Could you check a few things on this model? Use its own coordinates, in mm. A direction names the side the tool comes from. Coordinates: 2 decimals unless noted, no trailing zeros. Loops run counter-clockwise (first coordinate to the right, second up) from the corner with the lowest first, then second, coordinate; pieces in that order, holes last. Notation, with made-up numbers: M 60,80.25 L 111,80.25 A12 ccw 111,88.25 Z; hole C 3,-24 d2. An arc over 180 degrees is marked long. Write each question's results on one line, items separated by ' | '.
```python
from build123d import *

# Parameters (mm, degrees)
F1_DEPTH  = 40
F3_DEPTH  = 10
F4_W      = 20
F4_H      = 20
F5_DEPTH  = 20
F7_DEPTH  = 20
F9_DEPTH  = 20
F11_DEPTH = 20


with BuildPart() as f1:
    # F0 (on Front) → F1 (new body)
    with BuildSketch(Plane.XZ):
        Polygon((0, 40), (0, 0), (70, 0), (70, 20), (30, 20), (30, 40), align=None)
    extrude(amount=F1_DEPTH)

    # F2 (on face) → F3 (cut)
    with BuildSketch(Plane.XZ.offset(40)):
        Polygon((30, 20), (30, 40), (10, 40), align=None)
    extrude(amount=-F3_DEPTH, mode=Mode.SUBTRACT)

    # F4 (on face) → F5 (cut)
    with BuildSketch(Plane.XY.offset(40)):
        with Locations((20, -20)):
            Rectangle(F4_W, F4_H)
    extrude(amount=-F5_DEPTH, mode=Mode.SUBTRACT)

    # F6 (on face) → F7 (cut)
    with BuildSketch(Plane.XY.offset(20)):
        with BuildLine():
            ThreePointArc((60.3829629344, 0), (67.0878115757, -2.9325770906), (70, -9.6463064772))
            Line((70, -9.6463064772), (70, 0))
            Line((70, 0), (60.3829629344, 0))
        make_face()
    extrude(amount=-F7_DEPTH, mode=Mode.SUBTRACT)

    # F8 (on face) → F9 (cut)
    with BuildSketch(Plane.XY.offset(20)):
        with BuildLine():
            ThreePointArc((70, -32.718077302), (66.9100377104, -37.6307978482), (61.6119652987, -40))
            Line((61.6119652987, -40), (70, -40))
            Line((70, -40), (70, -32.718077302))
        make_face()
    extrude(amount=-F9_DEPTH, mode=Mode.SUBTRACT)

    # F10 (on face) → F11 (cut)
    with BuildSketch(Plane.XY.offset(20)):
        with BuildLine():
            ThreePointArc((50, -29.687499851), (57.0710678119, -26.7585676629), (60, -19.687499851))
            ThreePointArc((60, -19.687499851), (42.9289321881, -12.6164320391), (50, -29.687499851))
        make_face()
    extrude(amount=-F11_DEPTH, mode=Mode.SUBTRACT)


solid = f1.part
```
(1) Imagine slicing it at B-B, the plane y = -14. List the corners of the cut face in (x, z) for me, and give its area (3 significant figures).
Reported:
outline: M 0,0 L 41.77,0 L 41.77,20 L 10,20 L 10,40 L 0,40 Z; M 58.23,0 L 70,0 L 70,20 L 58.23,20 Z | area: 1,270 mm2
(2) If we mould it in two halves opening along Y, with no side actions, what happens to faces 1 (the flat face through (10, -20, 30)), 2 (the cylindrical face through (67.013, -2.859, 10.14)), 3 (the flat face through (35, -20, 0)), 4 (the cylindrical face through (66.97, -37.58, 10.14))? For each: released by +Y, released by -Y, zero draft, split by the parting line, or undercut.
Reported:
face 1: undercut | face 2: released by +Y | face 3: zero draft | face 4: released by -Y
(3) Please list where these lines run through material, in increasing order: probe 1 along Y at (x, z) = (50, 9.75); probe 2 along X at (y, z) = (-13, 38); probe 3 along Z at (x, y) = (32, -24.5). Write a range as from..to.
Reported:
probe 1: y = -40..-29.69, -9.69..0 | probe 2: x = 0..10 | probe 3: z = 0..20
(4) Imagine slicing it at A-A, the plane z = 10.5. List the corners of the cut face in (x, y) for me.
Reported:
outline: M 0,-40 L 61.61,-40 A10 ccw 70,-32.72 L 70,-9.65 A10 ccw 60.38,0 L 0,0 Z; hole C 50,-19.69 d20
(5) Will these pins go through, and if not, where does the flat tip stop? P1, Ø3, axis at x = 16.5, y = -14.5, coming from the +Z side; P2, Ø3, axis at y = -4, z = 32.5, coming from the +X side; P3, Ø10, axis at y = -17.5, z = 30, coming from the +X side.
Reported:
P1: stops at z = 20 | P2: stops at x = 30 | P3: stops at x = 10
(6) Imagine slicing it at D-D, the plane z = 34.5. List the corners of the cut face in (x, y) for me, and give its area (3 significant figures).
Reported:
outline: M 0,-40 L 15.5,-40 L 15.5,-30 L 10,-30 L 10,-10 L 30,-10 L 30,0 L 0,0 Z | area: 655 mm2
(7) Which directions (+Z, -Z, +X, -X, +Y, -Y) give clear straight access to the entire face, cutting with the end or side of a thin tool? Please do faces 5 (the flat face through (23, 0, 16)), 6 (the flat face through (30, -5, 30)), 7 (the flat face through (20, -35, 30)), 8 (the flat face through (15, -30, 26)).
Reported:
face 5: +Z, -Z, +X, -X, +Y | face 6: +Z, +X, +Y, -Y | face 7: +Z, +X, -Y | face 8: +Z, +X
(8) Imagine slicing it at C-C, the plane x = 18.5. List the corners of the cut face in (y, z) for me, and give its area (4 significant figures).
Reported:
outline: M -40,0 L 0,0 L 0,40 L -10,40 L -10,20 L -30,20 L -30,31.5 L -40,31.5 Z | area: 1,115 mm2
